```python
from build123d import *

# Parameters (mm, degrees)
SKETCH1_R           = 35
BOSS_EXTRUDE1_DEPTH = 32
SKETCH2_R           = 10
BOSS_EXTRUDE2_DEPTH = 5
CUT_EXTRUDE1_DEPTH  = 25
CUT_EXTRUDE2_DEPTH  = 36


with BuildPart() as part:
    # Sketch1 → Boss-Extrude1 (new body)
    with BuildSketch(Plane(origin=(0, 0, 0), x_dir=(1, 0, 0), z_dir=(0, 1, 0))):
        Circle(SKETCH1_R)
    extrude(amount=BOSS_EXTRUDE1_DEPTH)

    # Sketch2 → Boss-Extrude2 (add)
    with BuildSketch(Plane.XZ):
        Circle(SKETCH2_R)
    extrude(amount=BOSS_EXTRUDE2_DEPTH)

    # Sketch3 → Cut-Extrude1 (cut)
    with BuildSketch(Plane(origin=(0, 32, 0), x_dir=(1, 0, 0), z_dir=(0, 1, 0))):
        with BuildLine():
            Line((-9, 11), (9, 11))
            ThreePointArc((9, 11), (10.414213562, 10.414213562), (11, 9))
            Line((11, 9), (11, -9))
            ThreePointArc((11, -9), (10.414213562, -10.414213562), (9, -11))
            Line((9, -11), (-9, -11))
            ThreePointArc((-9, -11), (-10.414213562, -10.414213562), (-11, -9))
            Line((-11, -9), (-11, 9))
            ThreePointArc((-11, 9), (-10.414213562, 10.414213562), (-9, 11))
        make_face()
    extrude(amount=-CUT_EXTRUDE1_DEPTH, mode=Mode.SUBTRACT)

    # Sketch4 → Cut-Extrude2 (cut)
    with BuildSketch(Plane(origin=(0, 32, 0), x_dir=(1, 0, 0), z_dir=(0, 1, 0))):
        with BuildLine():
            Line((-1, 34.985711369), (-1, 33))
            Line((-1, 33), (1, 33))
            Line((1, 33), (1, 34.985711369))
            ThreePointArc((1, 34.985711369), (0, 35), (-1, 34.985711369))
        make_face()
        with BuildLine():
            Line((34.985711369, 1), (33, 1))
            Line((33, 1), (33, -1))
            Line((33, -1), (34.985711369, -1))
            ThreePointArc((34.985711369, -1), (35, 0), (34.985711369, 1))
        make_face()
        with BuildLine():
            Line((1, -34.985711369), (1, -33))
            Line((1, -33), (-1, -33))
            Line((-1, -33), (-1, -34.985711369))
            ThreePointArc((-1, -34.985711369), (0, -35), (1, -34.985711369))
        make_face()
        with BuildLine():
            Line((-34.985711369, -1), (-33, -1))
            Line((-33, -1), (-33, 1))
            Line((-33, 1), (-34.985711369, 1))
            ThreePointArc((-34.985711369, 1), (-35, 0), (-34.985711369, -1))
        make_face()
    extrude(amount=-CUT_EXTRUDE2_DEPTH, mode=Mode.SUBTRACT)


solid = part.part
```
Can you work these out from the model? Positions are in its coordinate system, mm. A direction names the side the tool comes from. Give positions to 0.01 mm unless a question says otherwise; leave off trailing zeros. Write each loop counter-clockwise with the first axis right and the second up, starting at its lowest first coordinate (ties: lowest second). Pieces come first, ordered by that corner, then holes. Notation, with made-up numbers: (65, 20) -> (90, 20) arc R25 cw to (90, 42) -> close; hole circle Ø11 at (8.25, 52.25). An arc over 180 degrees is marked (long way). One line per item, written item: value.
Q1. Imagine slicing it at A-A on y = 17.5. Please give me the cut outline in (x, z), and give its area (3 significant figures).
Results found:
outline: (-34.99, -1) arc R35 ccw to (-1, -34.99) -> (-1, -33) -> (1, -33) -> (1, -34.99) arc R35 ccw to (34.99, -1) -> (33, -1) -> (33, 1) -> (34.99, 1) arc R35 ccw to (1, 34.99) -> (1, 33) -> (-1, 33) -> (-1, 34.99) arc R35 ccw to (-34.99, 1) -> (-33, 1) -> (-33, -1) -> close; hole (-11, -9) arc R2 ccw to (-9, -11) -> (9, -11) arc R2 ccw to (11, -9) -> (11, 9) arc R2 ccw to (9, 11) -> (-9, 11) arc R2 ccw to (-11, 9) -> close
area: 3,350 mm^2
Q2. Please list where these lines run through material, in increasing order: line 1 (Y direction, x = -3.5, z = -7.5); line 2 (Y direction, x = 31, z = -7); line 3 (X direction, y = 15.5, z = -8). Write a range as [from, to].
Results found:
line 1: y = [-5, 7]
line 2: y = [0, 32]
line 3: x = [-34.07, -11], [11, 34.07]
Q3. Which directions (+Z, -Z, +X, -X, +Y, -Y) give clear straight access to the entire face, cutting with the end or side of a thin tool? Please do faces 4 (the face through (7.3, 0, 7.3)), 5 (the face through (0, 16, -33)), 6 (the face through (0, 7, 0)).
Results found:
face 4: -Y
face 5: -Z, +Y, -Y
face 6: +Y
Q4. Imagine slicing it at D-D on z = -28. Please give me the cut outline in (x, y), and give its area (3 significant figures).
Results found:
outline: (-21, 0) -> (21, 0) -> (21, 32) -> (-21, 32) -> close
area: 1,340 mm^2
Q5. Imagine slicing it at C-C on z = 0. Please give me the cut outline in (x, y), and give its area (3 significant figures).
Results found:
outline: (-33, 0) -> (-10, 0) -> (-10, -5) -> (10, -5) -> (10, 0) -> (33, 0) -> (33, 32) -> (11, 32) -> (11, 7) -> (-11, 7) -> (-11, 32) -> (-33, 32) -> close
area: 1,660 mm^2
Q6. Imagine slicing it at B-B on x = 0. Please give me the cut outline in (y, z).
Results found:
outline: (-5, -10) -> (0, -10) -> (0, -33) -> (32, -33) -> (32, -11) -> (7, -11) -> (7, 11) -> (32, 11) -> (32, 33) -> (0, 33) -> (0, 10) -> (-5, 10) -> close
Q7. For P1, Ø1, axis at x = 18, y = 9.5, coming from the +Z side; P2, Ø1, axis at x = -8, z = 19.5, coming from the -Y side; P3, Ø6, axis at x = 23, y = 6.5, coming from the +Z side; P4, Ø24, axis at x = 4.5, z = -1.5, coming from the +Y side, each with a flat end and sliding along its axis, tell me the tip position at first contact or that it passes through.
Results found:
P1: stops at z = 30.31
P2: stops at y = 0
P3: stops at z = 28.72
P4: stops at y = 32
Q8. We'd pull the mould along X, two halves only. Please class faces 1 (the face through (34, 16, 1)), 2 (the face through (33, 16, 0)), 3 (the face through (-10.43, 19.68, -10.4)): +X half, -X half, draft (parallel to the pull), parting line (faces both ways), or undercut.
Results found:
face 1: draft
face 2: +X half
face 3: undercut
